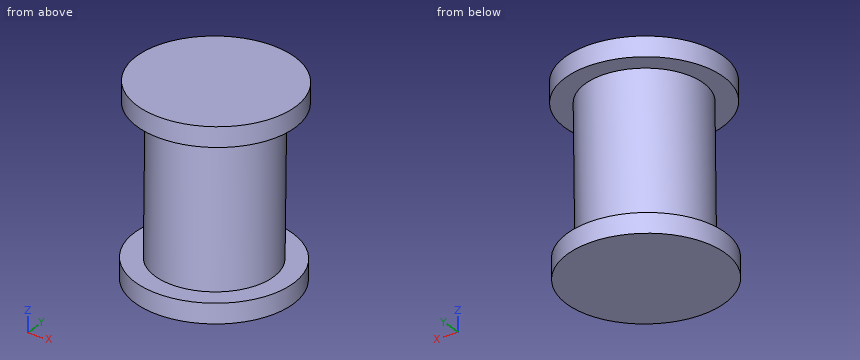
```python
from build123d import *

# Parameters (mm, degrees)
BODY_MOVE_COPY1_ANGLE = 119.424338974


with BuildPart() as part:
    # Sketch1 → Revolve1 (revolve)
    with BuildSketch(Plane.XY, mode=Mode.PRIVATE) as revolve1_sk:
        Polygon((0, 0), (0, 9.5), (-4, 9.5), (-4, 8.5), (-3, 8.5), (-3, 1), (-4, 1), (-4, 0), align=None)
    revolve(revolve1_sk.sketch.rotate(Axis((0, 0, 0), (0, 1, 0)), 270), axis=Axis((0, 0, 0), (0, 1, 0)))


with BuildPart() as part_1:
    # Body-Move/Copy1: moved
    add(part.part.moved(Location((0, 0, 0))).rotate(Axis((-2.346629399, 4.612052575, -2.346629399), (0.5739619558891293, 0.5840679295973761, 0.5739619558888548)), BODY_MOVE_COPY1_ANGLE))


solid = part_1.part
```
Can you work these out from the model? Positions are in its coordinate system, mm. Give positions to 0.01 mm unless a question says otherwise; leave off trailing zeros. Write each loop counter-clockwise with the first axis right and the second up, starting at its lowest first coordinate (ties: lowest second). Pieces come first, ordered by that corner, then holes. Notation, with made-up numbers: (66, -36.5) - (108, -36.5) arc R17 ccw to (108, -10.5) - close; hole circle Ø7 at (23, 48.25). An arc over 180 degrees is marked (long way). Write item = value, one per line. Start each with the question number.
1. For pin 1 (3 mm diameter, centred on y = 4.5, z = -1, fed in from -X); pin 2 (3 mm diameter, centred on x = -2, z = -1, fed in from -Y); pin 3 (1.5 mm diameter, centred on x = -3, z = -4.5, fed in from -Y), each with a flat end and sliding along its axis, tell me the tip position at first contact or that it passes through.
2. Imagine slicing it at C-C (x = 1). Please give me the cut outline in (y, z).
3. Imagine slicing it at A-A (x = 3.25). Please give me the cut outline in (y, z).
4. Please list where these lines run through material, in increasing order: line 1 (Z direction, x = 1.25, y = 10.5); line 2 (Y direction, x = -2.5, z = -1.5); line 3 (Z direction, x = 3, y = 5.75).
5. Imagine slicing it at B-B (x = -0.25). Please give me the cut outline in (y, z), and give its area (3 significant figures).
Worked answers:
q1.pin_1 = -2.83
q1.pin_2 = 4.02
q1.pin_3 = 4.94
q2.outline = (3.01, -6.93) - (10.75, -7.07) - (10.77, -6.07) - (9.72, -6.05) - (9.85, 1.45) - (10.9, 1.43) - (10.92, 2.43) - (3.17, 2.57) - (3.15, 1.57) - (4.2, 1.55) - (4.07, -5.95) - (3.02, -5.93) - close
q3.outline = (4.55, -6.96) - (9.21, -7.04) - (9.23, -6.04) - (4.56, -5.96) - close; (4.69, 1.54) - (9.36, 1.46) - (9.38, 2.46) - (4.71, 2.54) - close
q4.line_1 = -7.06 to -6.06, 1.44 to 2.44
q4.line_2 = 5.32 to 8.63
q4.line_3 = -6.98 to -5.98, 1.52 to 2.52
q5.outline = (2.89, -6.93) - (10.87, -7.07) - (10.89, -6.07) - (9.88, -6.05) - (10.02, 1.45) - (11.02, 1.43) - (11.04, 2.43) - (3.05, 2.57) - (3.03, 1.57) - (4.04, 1.55) - (3.91, -5.95) - (2.9, -5.93) - close
q5.area = 60.8 mm2
